The listing builds one solid part. Answer for the finished solid, in the listing's coordinates (mm). A direction names the side the tool comes from. Round coordinates to 2 decimals unless told otherwise and drop trailing zeros. Write each loop counter-clockwise with the first axis right and the second up, starting at its lowest first coordinate (ties: lowest second). Pieces come first, ordered by that corner, then holes.
(1) A cutting plane is placed at B-B, the plane z = 3. Give the vertices of the cut face in (x, y), and give its area (3 significant figures).
(2) A cutting plane is placed at D-D, the plane z = -37.5. Give the vertices of the cut face in (x, y), and give its area (3 significant figures).
(3) This flat-tipped pin is pushed along its axis until it touches: pin 1 Ø4 at (x, z) = (-6, -28.5) entering from +Y. Where does it stop, or does it pass through?
(4) A cutting plane is placed at C-C, the plane y = -8.5. Give the vertices of the cut face in (x, z), and give its area (4 significant figures).
(5) The mould has two halves that part along Y. Classify faces 1 (the face through (1, -25, -1)), 2 (the face through (15, -11.708, 0)), 3 (the face through (-9.849, -12, -1)): +Y half, -Y half, draft (parallel to the pull), parting line (faces both ways), or undercut.
(6) A cutting plane is placed at A-A, the plane y = -16.75. Give the vertices of the cut face in (x, z), and give its area (4 significant figures).
(7) Find the intervals of material crossed by probe 1 along X at (y, z) = (-5.25, 10.5); probe 2 along Y at (x, z) = (-5.5, 44.5); probe 3 along Z at (x, y) = (-1.5, -7.25), in increasing order.
(8) For faces 4 (the face through (-10, 0, 4)), 5 (the face through (12.651, -10, -1)), 6 (the face through (15, -16, -9.839)), determine the directions among +Z, -Z, +X, -X, +Y, -Y from which every point of the face is accessible in a straight line to the end or side of a thin tool.
from build123d import *

# Parameters (mm, degrees)
BOSS_EXTRUDE1_DEPTH = 50
SKETCH2_W           = 30.5
SKETCH2_H           = 29
BOSS_EXTRUDE2_DEPTH = 3
SKETCH3_W           = 19.5
SKETCH3_H           = 8.69
CUT_EXTRUDE1_DEPTH  = 30


with BuildPart() as part:
    # Sketch1 → Boss-Extrude1 (new body, symmetric)
    with BuildSketch(Plane.XY):
        Polygon((-9.848648649, 0), (-9.848648649, -25), (12.651351351, -25), (12.651351351, 0), (16.651351351, 0), (16.651351351, -29), (-13.848648649, -29), (-13.848648649, 0), align=None)
    extrude(amount=BOSS_EXTRUDE1_DEPTH, both=True)

    # Sketch2 → Boss-Extrude2 (add)
    with BuildSketch(Plane.XY.offset(50)):
        with Locations((1.401351351, -14.5)):
            Rectangle(SKETCH2_W, SKETCH2_H)
    extrude(amount=-BOSS_EXTRUDE2_DEPTH)

    # Sketch3 → Cut-Extrude1 (cut)
    with BuildSketch(Plane(origin=(0, 0, 0), x_dir=(0, 0, -1), z_dir=(1, 0, 0))):
        with Locations((0.088778278, -16.052995557)):
            Rectangle(SKETCH3_W, SKETCH3_H)
    extrude(amount=CUT_EXTRUDE1_DEPTH, mode=Mode.SUBTRACT)


solid = part.part
Solutions:
1. outline: (-13.85, -29) - (16.65, -29) - (16.65, -20.4) - (12.65, -20.4) - (12.65, -25) - (-9.85, -25) - (-9.85, 0) - (-13.85, 0) - close; (12.65, -11.71) - (16.65, -11.71) - (16.65, 0) - (12.65, 0) - close
1. area: 287 mm2
2. outline: (-13.85, -29) - (16.65, -29) - (16.65, 0) - (12.65, 0) - (12.65, -25) - (-9.85, -25) - (-9.85, 0) - (-13.85, 0) - close
2. area: 322 mm2
3. pin 1: stops at y = -25
4. outline: (-13.85, -50) - (-9.85, -50) - (-9.85, 47) - (12.65, 47) - (12.65, -50) - (16.65, -50) - (16.65, 50) - (-13.85, 50) - close
4. area: 867.5 mm2
5. face 1: +Y half
5. face 2: undercut
5. face 3: draft
6. outline: (-13.85, -50) - (-9.85, -50) - (-9.85, 47) - (12.65, 47) - (12.65, 9.66) - (16.65, 9.66) - (16.65, 50) - (-13.85, 50) - close; (12.65, -50) - (16.65, -50) - (16.65, -9.84) - (12.65, -9.84) - close
6. area: 789.5 mm2
7. probe 1: x = -13.85 to -9.85, 12.65 to 16.65
7. probe 2: y = -29 to -25
7. probe 3: z = 47 to 50
8. face 4: +Z, -Z, +X, -X, +Y
8. face 5: -Z, +Y
8. face 6: +X
